Check sheet for the modelled part. Datum: model origin and axes. Units: mm. Give positions to 0.01 mm unless a question says otherwise; leave off trailing zeros. Loops run counter-clockwise (first coordinate to the right, second up) from the corner with the lowest first, then second, coordinate; pieces in that order, holes last. Notation, with made-up numbers: M 39.5,-5.75 L 49.5,-5.75 A16 cw 49.5,18.25 Z; hole C -4.5,39.5 d2. An arc over 180 degrees is marked long. Use one line per item in the form item = value.
from build123d import *

# Parameters (mm, degrees)
SKETCH1_R               = 7.94
SKETCH1_R_2             = 6.44
BOSS_EXTRUDE1_DEPTH     = 49.82
CHAMFER1_SIZE           = 0.25
SKETCH2_R               = 1.55
CUT_EXTRUDE1_DEPTH      = 53.299522942
CUT_EXTRUDE1_DEPTH_BACK = 53.299522942


with BuildPart() as part:
    # Sketch1 → Boss-Extrude1 (new body)
    with BuildSketch(Plane(origin=(0, 0, 0), x_dir=(1, 0, 0), z_dir=(0, 1, 0))):
        with Locations(Location((0, 0, 0), (0, 0, 270))):
            Circle(SKETCH1_R)
        with Locations(Location((0, 0, 0), (0, 0, 270))):
            Circle(SKETCH1_R_2, mode=Mode.SUBTRACT)
    extrude(amount=BOSS_EXTRUDE1_DEPTH)

    # Chamfer1
    chamfer1_edges = [part.edges().sort_by_distance(p)[0] for p in [
        (0, 0, -7.94),
        (0, 49.82, -7.94),
    ]]
    chamfer(chamfer1_edges, length=CHAMFER1_SIZE)

    # Sketch2 → Cut-Extrude1 (cut, two sides)
    with BuildSketch(Plane(origin=(0, 0, -5.85), x_dir=(-1, 0, 0), z_dir=(0, 0, -1))) as cut_extrude1_sk:
        with Locations((0.000190227, 7.5)):
            Circle(SKETCH2_R)
        with BuildLine():
            add(Edge.make_bspline(
                [(1.550190227, 42.32), (1.550190227, 45.42), (-1.549809773, 45.42), (-1.549809773, 42.32), (-1.549809773, 39.22), (1.550190227, 39.22), (1.550190227, 42.32)],
                knots=[0, 0, 0, 0, 0.5, 0.5, 0.5, 1, 1, 1, 1], degree=3, weights=[1, 0.333333333, 0.333333333, 1, 0.333333333, 0.333333333, 1]))
        make_face()
    extrude(amount=CUT_EXTRUDE1_DEPTH, mode=Mode.SUBTRACT)
    extrude(cut_extrude1_sk.sketch, amount=-CUT_EXTRUDE1_DEPTH_BACK, mode=Mode.SUBTRACT)


solid = part.part
1) Release check for a two-part mould opening along Z. For faces 1 (the face through (-5, 0, -5)), 2 (the face through (2.385, 24.565, 7.573)), 3 (the face through (-2.467, 24.561, 5.949)) record: pulls with the +Z half, pulls with the -Z half, needs draft (parallel to the pull), parting line crosses it, or undercut.
Evaluation:
face_1 = needs draft
face_2 = parting line crosses it
face_3 = undercut
2) Scan lines: line 1 (Z direction, x = 0, y = 20.5); line 2 (Z direction, x = 2, y = 35). Record each from-to range of solid material in increasing order.
Evaluation:
line_1 = -7.94 to -6.44, 6.44 to 7.94
line_2 = -7.68 to -6.12, 6.12 to 7.68
3) Section check C-C (x = 0). State how many separate pieces and enclosed holes the cut face has, then the cut area to 3 significant figures.
Evaluation:
separate_pieces = 6
enclosed_holes = 0
area = 131 mm^2
4) Depth check by flat-ended pin: pin 1 Ø2 at (y, z) = (19.5, 2.5) entering from -X; pin 2 Ø3 at (x, y) = (5.5, 32.5) entering from +Z. Enter the tip coordinate at first touch or a pass-through.
Evaluation:
pin_1 = -7.8
pin_2 = 6.86
5) Section check A-A (z = 0). Record the cut outline in (x, y).
Evaluation:
outline = M -7.94,0.25 L -7.69,0 L -6.44,0 L -6.44,49.82 L -7.69,49.82 L -7.94,49.57 Z; M 6.44,0 L 7.69,0 L 7.94,0.25 L 7.94,49.57 L 7.69,49.82 L 6.44,49.82 Z
6) Section check B-B (y = 7.5). Record the cut outline in (x, z), then the cut area to 3 significant figures.
Evaluation:
outline = M -1.55,-7.79 L -1.55,-6.25 A6.44 cw -1.55,6.25 L -1.55,7.79 A7.94 ccw Z; M 1.55,-7.79 A7.94 ccw 1.55,7.79 L 1.55,6.25 A6.44 cw 1.55,-6.25 Z
area = 58.4 mm^2
7) Section check D-D (y = 35). Record the cut outline in (x, z).
Evaluation:
outline = C 0,0 d15.88; hole C 0,0 d12.88
